Geometry: final body of the model. Coordinates: model frame, mm. A direction names the side the tool comes from. Coordinates: 2 decimals unless noted, no trailing zeros. Order: outer loops, then holes, each group sorted by start corner. A loop starts at its lowest first (then second) coordinate and runs counter-clockwise, first axis right, second up. Notation, with made-up numbers: M -1,-39 L 6,-39 A19 ccw 6,-15 Z; hole C -37.5,-10 d3. An arc over 180 degrees is marked long. Use CSV: the item, a comma, the result in double quotes. Start each with the question number.
1. Section query C-C on x = 7.5. Return the cut outline in (y, z).
2. Section query D-D on y = 0. State how many separate pieces and enclosed holes the cut face has, and give its area (3 significant figures).
3. Section query A-A on y = -76.2. Return the cut outline in (x, z) (3 decimals), and give its area (3 significant figures).
4. Pull-direction query (Y, two-part tool) for faces 3 (the flat face through (9.525, 20, -1)), 4 (the cylindrical face through (4.696, 92.985, -20.648)), 5 (the cylindrical face through (4.696, 0.517, -72.265)); classes: pulls with the +Y half, pulls with the -Y half, needs draft (parallel to the pull), parting line crosses it, or undercut.
5. Set-up query: faces 1 (the cylindrical face through (7.18, -12.4, 2.75)), 2 (the cylindrical face through (4.696, -72.265, -0.517)). Return all of +Z, -Z, +X, -X, +Y, -Y with unobstructed straight access to the full face (end or side cutting, diameter ignored); none if empty.
6. Material intervals for line 1 (Y direction, x = 7, z = 0); line 2 (Y direction, x = 3.5, z = 0); line 3 (Z direction, x = 4.75, y = 76.2), sorted ascending.
7. First-contact query: P1, Ø10.5, axis at y = 0, z = 76.2, coming from the -X side; P2, Ø5, axis at x = 4.5, z = -32.5, coming from the +Y side; P3, Ø1.5, axis at x = 2, y = 46.5, coming from the -Z side; P4, Ø5, axis at y = -76.2, z = 0, coming from the +X side. Flat tips, straight axial feed; report the tip coordinate or a pass-through.
from build123d import *

# Parameters (mm, degrees)
SKETCH1_R               = 95.25
BOSS_EXTRUDE1_DEPTH     = 9.525
SKETCH2_R               = 12.7
CUT_EXTRUDE1_DEPTH      = 4.7625
F_3_8_16_TAPPED_HOLE1_D = 7.9375
CIRPATTERN1_COUNT       = 4


with BuildPart() as part:
    # Sketch1 → Boss-Extrude1 (new body)
    with BuildSketch(Plane(origin=(0, 0, 0), x_dir=(0, 0, -1), z_dir=(1, 0, 0))):
        with Locations(Location((0, 0, 0), (0, 0, 180))):
            Circle(SKETCH1_R)
    extrude(amount=BOSS_EXTRUDE1_DEPTH)

    # Sketch2 → Cut-Extrude1 (cut)
    with BuildSketch(Plane(origin=(9.525, 0, 0), x_dir=(0, 0, -1), z_dir=(1, 0, 0))):
        Circle(SKETCH2_R)
    extrude(amount=-CUT_EXTRUDE1_DEPTH, mode=Mode.SUBTRACT)

    # Sketch4 → CSK for 1/2 Flat Head Machine Screw1 (revolve, cut)
    with BuildSketch(Plane.ZX):
        Polygon((0, 0), (0, 9.525), (6.74624, 9.525), (6.74624, 5.022807562), (11.1125, 0), align=None)
    revolve(axis=Axis((-6.35, 0, 0), (1, 0, 0)), mode=Mode.SUBTRACT)

    # 3/8-16 Tapped Hole1 (through all)
    with Locations(Plane(origin=(9.525, 0, 0), x_dir=(0, 0, -1), z_dir=(1, 0, 0))):
        with Locations((0, -76.2)):
            f_3_8_16_tapped_hole1 = Hole(F_3_8_16_TAPPED_HOLE1_D / 2)

    # CirPattern1: 3/8-16 Tapped Hole1 ×4 about axis
    cirpattern1_axis = Axis((0, 0, 0), (1, 0, 0))
    for i in range(1, CIRPATTERN1_COUNT):
        add(f_3_8_16_tapped_hole1.rotate(cirpattern1_axis, i * 360 / CIRPATTERN1_COUNT), mode=Mode.SUBTRACT)


solid = part.part
Results list:
1,outline,"C 0,0 d190.5; hole C -76.2,0 d7.94; hole C 0,0 d25.4; hole C 0,-76.2 d7.94; hole C 0,76.2 d7.94; hole C 76.2,0 d7.94"
2,separate pieces,"4"
2,enclosed holes,"0"
2,area,"1,460 mm²"
3,outline,"M 0,-57.15 L 9.525,-57.15 L 9.525,-3.969 L 0,-3.969 Z; M 0,3.969 L 9.525,3.969 L 9.525,57.15 L 0,57.15 Z"
3,area,"1,010 mm²"
4,face 3,"needs draft"
4,face 4,"parting line crosses it"
4,face 5,"undercut"
5,face 1,"+X"
5,face 2,"+X, -X"
6,line 1,"y = -95.25 to -80.17, -72.23 to -12.7, 12.7 to 72.23, 80.17 to 95.25"
6,line 2,"y = -95.25 to -80.17, -72.23 to -8.07, 8.07 to 72.23, 80.17 to 95.25"
6,line 3,"z = -57.15 to -3.97, 3.97 to 57.15"
7,P1,"stops at x = 0"
7,P2,"stops at y = 90.4"
7,P3,"stops at z = -83.54"
7,P4,"passes through"
